Here's how the part is built. I have some questions about the finished solid (model axes, mm). A direction names the side the tool comes from. Round coordinates to 2 decimals unless told otherwise and drop trailing zeros. Write each loop counter-clockwise with the first axis right and the second up, starting at its lowest first coordinate (ties: lowest second). Pieces come first, ordered by that corner, then holes. Notation, with made-up numbers: (-6.5, 28.5) -> (19.5, 28.5) arc R31 ccw to (19.5, 54.5) -> close; hole circle Ø10 at (87, -39). An arc over 180 degrees is marked (long way). Answer as CSV lines item,"result".
from build123d import *

# Parameters (mm, degrees)
ESBO_O1_W                = 247
ESBO_O1_H                = 150
RESSALTO_EXTRUS_O1_DEPTH = 55
FILETE1_R                = 5
FILETE2_R                = 3
CASCA1_T                 = -4


with BuildPart() as part:
    # Esboço1 → Ressalto-extrusão1 (new body)
    with BuildSketch(Plane(origin=(0, 0, 0), x_dir=(1, 0, 0), z_dir=(0, 1, 0))):
        Rectangle(ESBO_O1_W, ESBO_O1_H)
    extrude(amount=RESSALTO_EXTRUS_O1_DEPTH)

    # Filete1
    filete1_edges = [part.edges().sort_by_distance(p)[0] for p in [
        (123.5, 27.5, 75),
        (-123.5, 27.5, 75),
        (-123.5, 27.5, -75),
        (123.5, 27.5, -75),
    ]]
    fillet(filete1_edges, radius=FILETE1_R)

    # Filete2
    filete2_edges = [part.edges().sort_by_distance(p)[0] for p in [
        (-123.5, 0, 0),
        (123.5, 0, 0),
        (0, 0, 75),
        (0, 0, -75),
        (122.035533906, 0, 73.535533906),
        (122.035533906, 0, -73.535533906),
        (-122.035533906, 0, 73.535533906),
        (-122.035533906, 0, -73.535533906),
    ]]
    fillet(filete2_edges, radius=FILETE2_R)

    # Casca1
    casca1_openings = [part.faces().sort_by_distance(p)[0] for p in [
        (0, 55, 0),
    ]]
    offset(amount=CASCA1_T, openings=casca1_openings, kind=Kind.INTERSECTION)


solid = part.part
Item 1: Will this pin go through, and if not, where does the flat tip stop? pin 1 (2 mm diameter, centred on x = -78, z = 46.5, fed in from +Y).
Results found:
pin 1,"stops at y = 4"
Item 2: Suppose I cut it at B-B, the plane x = -2.5. List the corners of the cut face in (y, z) for me, then the cut area to 3 significant figures.
Results found:
outline,"(0, -72) arc R3 ccw to (3, -75) -> (55, -75) -> (55, -71) -> (4, -71) -> (4, 71) -> (55, 71) -> (55, 75) -> (3, 75) arc R3 ccw to (0, 72) -> close"
area,"1,000 mm²"
Item 3: Suppose I cut it at C-C, the plane z = 16. List the corners of the cut face in (x, y) for me, then the cut area to 3 significant figures.
Results found:
outline,"(-123.5, 3) arc R3 ccw to (-120.5, 0) -> (120.5, 0) arc R3 ccw to (123.5, 3) -> (123.5, 55) -> (119.5, 55) -> (119.5, 4) -> (-119.5, 4) -> (-119.5, 55) -> (-123.5, 55) -> close"
area,"1,390 mm²"
Item 4: If we mould it in two halves opening along Z, with no side actions, what happens to faces 1 (the flat face through (-2, 29, -75)), 2 (the cylindrical face through (-122.07, 29.36, 73.5)), 3 (the flat face through (-119.5, 29, 1))? For each: pulls with the +Z half, pulls with the -Z half, needs draft (parallel to the pull), parting line crosses it, or undercut.
Results found:
face 1,"pulls with the -Z half"
face 2,"pulls with the +Z half"
face 3,"undercut"
Item 5: For faces 4 (the flat face through (-2, 29, -71)), 5 (the cylindrical face through (122.07, 29.36, -73.5)), which set-ups out of +Z, -Z, +X, -X, +Y, -Y let a thin tool reach every point of the face, with its end or its side?
Results found:
face 4,"+Y"
face 5,"-Z, +X, +Y, -Y"
Item 6: Suppose I cut it at A-A, the plane y = 35. List the corners of the cut face in (x, z) for me.
Results found:
outline,"(-123.5, -70) arc R5 ccw to (-118.5, -75) -> (118.5, -75) arc R5 ccw to (123.5, -70) -> (123.5, 70) arc R5 ccw to (118.5, 75) -> (-118.5, 75) arc R5 ccw to (-123.5, 70) -> close; hole (-119.5, -70) arc R1 ccw to (-118.5, -71) -> (118.5, -71) arc R1 ccw to (119.5, -70) -> (119.5, 70) arc R1 ccw to (118.5, 71) -> (-118.5, 71) arc R1 ccw to (-119.5, 70) -> close"
Item 7: I need wall thicknesses on L1, parallel to Z at x = -72, y = 31.5; L2, parallel to X at y = 51.5, z = 42; L3, parallel to Y at x = -105.5, z = -2.5. Which ranges of each line are inside material? Lowest first, please.
Results found:
L1,"z = -75 to -71, 71 to 75"
L2,"x = -123.5 to -119.5, 119.5 to 123.5"
L3,"y = 0 to 4"
